Geometry check sheet. Reference: the model listing, model coordinates, mm. Face numbers are marked on the shaded views. A direction names the side the tool comes from. Coordinates: 2 decimals unless noted, no trailing zeros. Loops run counter-clockwise (first coordinate to the right, second up) from the corner with the lowest first, then second, coordinate; pieces in that order, holes last.
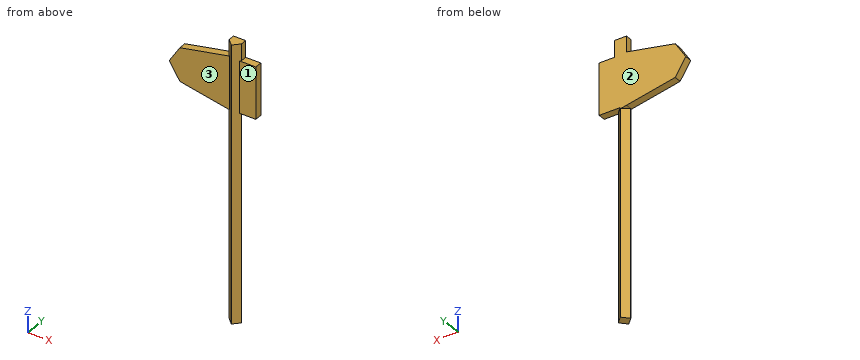
from build123d import *

# Parameters (mm, degrees)
F0_W         = 10.6080286205
F0_H         = 181.0148730874
F1_DEPTH     = 10.52446
F0_W_2       = 13.1920464337
F0_H_2       = 45.1798141003
F2_DEPTH     = 6.38094
F3_T1_DEPTH  = 194.0790226663
F3_T6_DEPTH  = 266.8450713117
F3_T12_DEPTH = 266.8450713117
F3_T18_DEPTH = 266.8450713117
F3_T25_DEPTH = 266.8450713117
F3_T31_DEPTH = 266.8450713117
F3_T37_DEPTH = 266.8450713117
F3_T43_DEPTH = 266.8450713117
F3_T49_DEPTH = 266.8450713117
F3_T56_DEPTH = 266.8450713117
F3_T62_DEPTH = 266.8450713117
F3_T68_DEPTH = 207.1431722451


# Not quite as in the source:
# - a fillet or chamfer that OpenCascade refuses, or shapes differently, is made with other operations: its cross-section is extruded or revolved along the edge and cut away or added


with BuildPart() as f1:
    # F0 (on Front) → F1 (new body)
    with BuildSketch(Plane.XZ):
        with Locations((36.9313266128, -119.8917590082)):
            Rectangle(F0_W, F0_H)
        Polygon((42.2353409231, 15.7954916358), (42.2353409231, 30.3175766021), (31.6273123026, 30.3175766021), (31.6273123026, 16.6022777557), align=None)
        Polygon((42.2353409231, -29.3843224645), (42.2353409231, 15.7954916358), (31.6273123026, 16.6022777557), (31.6273123026, -29.3843224645), align=None)
    extrude(amount=F1_DEPTH)

    # F0 (on Front) → F2 (join)
    with BuildSketch(Plane.XZ):
        Polygon((42.2353409231, 15.7954916358), (42.2353409231, 30.3175766021), (31.6273123026, 30.3175766021), (31.6273123026, 16.6022777557), align=None)
        with Locations((48.8313641399, -6.7944154143)):
            Rectangle(F0_W_2, F0_H_2)
        Polygon((42.2353409231, -29.3843224645), (42.2353409231, 15.7954916358), (31.6273123026, 16.6022777557), (31.6273123026, -29.3843224645), align=None)
        with Locations((36.9313266128, -119.8917590082)):
            Rectangle(F0_W, F0_H)
        Polygon((31.6273123026, -29.3843224645), (31.6273123026, 16.6022777557), (-10.7287643477, 8.1310607493), (-20.0067628175, -6.3910223544), (-10.7287643477, -20.913105458), align=None)
    extrude(amount=F2_DEPTH)

    # F3: chamfer of 5.08 on 4 edges, made by hand

    # F3_s2 → F3_t1 (cut)
    with BuildSketch(Plane.XY.offset(-223.4633451307)):
        Polygon((42.2353409231, -5.08), (37.1553409231, 0), (42.2353409231, 0), align=None)
    extrude(amount=F3_T1_DEPTH, mode=Mode.SUBTRACT)


with BuildPart() as f3_tool4:
    # F3_s5 → F3_t6 (new body)
    with BuildSketch(Plane.XY.offset(-223.4633451307)):
        Polygon((42.2353409231, -5.44446), (37.1553409231, -10.52446), (42.2353409231, -10.52446), align=None)
    extrude(amount=F3_T6_DEPTH)

    split(bisect_by=Plane.XZ.offset(6.38094), keep=Keep.BOTTOM)

    split(bisect_by=Plane.XY.offset(-29.3843224645), keep=Keep.BOTTOM)


with BuildPart() as f1_1:
    add(f1.part)

    # F3_t3: cut F3_tool4
    add(f3_tool4.part, mode=Mode.SUBTRACT)


with BuildPart() as f3_tool10:
    # F3_s11 → F3_t12 (new body)
    with BuildSketch(Plane.XY.offset(-223.4633451307)):
        Polygon((42.2353409231, -5.44446), (37.1553409231, -10.52446), (42.2353409231, -10.52446), align=None)
    extrude(amount=F3_T12_DEPTH)

    split(bisect_by=Plane.XZ.offset(6.38094), keep=Keep.TOP)

    split(bisect_by=Plane.XY.offset(-29.3843224645), keep=Keep.BOTTOM)


with BuildPart() as f1_2:
    add(f1_1.part)

    # F3_t9: cut F3_tool10
    add(f3_tool10.part, mode=Mode.SUBTRACT)


with BuildPart() as f3_tool16:
    # F3_s17 → F3_t18 (new body)
    with BuildSketch(Plane.XY.offset(-223.4633451307)):
        Polygon((42.2353409231, -5.44446), (37.1553409231, -10.52446), (42.2353409231, -10.52446), align=None)
    extrude(amount=F3_T18_DEPTH)

    split(bisect_by=Plane.XY.offset(15.7954916358), keep=Keep.BOTTOM)

    split(bisect_by=Plane.XZ.offset(6.38094), keep=Keep.TOP)

    split(bisect_by=Plane.XY.offset(-29.3843224645), keep=Keep.TOP)


with BuildPart() as f1_3:
    add(f1_2.part)

    # F3_t15: cut F3_tool16
    add(f3_tool16.part, mode=Mode.SUBTRACT)


with BuildPart() as f3_tool23:
    # F3_s24 → F3_t25 (new body)
    with BuildSketch(Plane.XY.offset(-223.4633451307)):
        Polygon((42.2353409231, -5.44446), (37.1553409231, -10.52446), (42.2353409231, -10.52446), align=None)
    extrude(amount=F3_T25_DEPTH)

    split(bisect_by=Plane.XY.offset(15.7954916358), keep=Keep.TOP)

    split(bisect_by=Plane.XZ.offset(6.38094), keep=Keep.BOTTOM)


with BuildPart() as f1_4:
    add(f1_3.part)

    # F3_t22: cut F3_tool23
    add(f3_tool23.part, mode=Mode.SUBTRACT)


with BuildPart() as f3_tool29:
    # F3_s30 → F3_t31 (new body)
    with BuildSketch(Plane.XY.offset(-223.4633451307)):
        Polygon((42.2353409231, -5.44446), (37.1553409231, -10.52446), (42.2353409231, -10.52446), align=None)
    extrude(amount=F3_T31_DEPTH)

    split(bisect_by=Plane.XY.offset(15.7954916358), keep=Keep.TOP)

    split(bisect_by=Plane.XZ.offset(6.38094), keep=Keep.TOP)


with BuildPart() as f1_5:
    add(f1_4.part)

    # F3_t28: cut F3_tool29
    add(f3_tool29.part, mode=Mode.SUBTRACT)


with BuildPart() as f3_tool35:
    # F3_s36 → F3_t37 (new body)
    with BuildSketch(Plane.XY.offset(43.381726181)):
        Polygon((31.6273123026, -5.44446), (36.7073123026, -10.52446), (31.6273123026, -10.52446), align=None)
    extrude(amount=-F3_T37_DEPTH)

    split(bisect_by=Plane.XZ.offset(6.38094), keep=Keep.BOTTOM)

    split(bisect_by=Plane(origin=(-1.976310754, 0, 9.8815518144), x_dir=(0, 1, 0), z_dir=(-0.1961161725, 0, 0.9805806682)), keep=Keep.TOP)


with BuildPart() as f1_6:
    add(f1_5.part)

    # F3_t34: cut F3_tool35
    add(f3_tool35.part, mode=Mode.SUBTRACT)


with BuildPart() as f3_tool41:
    # F3_s42 → F3_t43 (new body)
    with BuildSketch(Plane.XY.offset(43.381726181)):
        Polygon((31.6273123026, -5.44446), (36.7073123026, -10.52446), (31.6273123026, -10.52446), align=None)
    extrude(amount=-F3_T43_DEPTH)

    split(bisect_by=Plane.XZ.offset(6.38094), keep=Keep.TOP)

    split(bisect_by=Plane(origin=(-1.976310754, 0, 9.8815518144), x_dir=(0, 1, 0), z_dir=(-0.1961161725, 0, 0.9805806682)), keep=Keep.TOP)


with BuildPart() as f1_7:
    add(f1_6.part)

    # F3_t40: cut F3_tool41
    add(f3_tool41.part, mode=Mode.SUBTRACT)


with BuildPart() as f3_tool47:
    # F3_s48 → F3_t49 (new body)
    with BuildSketch(Plane.XY.offset(43.381726181)):
        Polygon((31.6273123026, -5.44446), (36.7073123026, -10.52446), (31.6273123026, -10.52446), align=None)
    extrude(amount=-F3_T49_DEPTH)

    split(bisect_by=Plane(origin=(-4.4343967239, 0, -22.1719792319), x_dir=(0, 1, 0), z_dir=(0.1961161725, 0, 0.9805806682)), keep=Keep.TOP)

    split(bisect_by=Plane.XZ.offset(6.38094), keep=Keep.TOP)

    split(bisect_by=Plane(origin=(-1.976310754, 0, 9.8815518144), x_dir=(0, 1, 0), z_dir=(0.1961161725, 0, -0.9805806682)), keep=Keep.TOP)


with BuildPart() as f1_8:
    add(f1_7.part)

    # F3_t46: cut F3_tool47
    add(f3_tool47.part, mode=Mode.SUBTRACT)


with BuildPart() as f3_tool54:
    # F3_s55 → F3_t56 (new body)
    with BuildSketch(Plane.XY.offset(43.381726181)):
        Polygon((31.6273123026, -5.44446), (36.7073123026, -10.52446), (31.6273123026, -10.52446), align=None)
    extrude(amount=-F3_T56_DEPTH)

    split(bisect_by=Plane(origin=(-4.4343967239, 0, -22.1719792319), x_dir=(0, 1, 0), z_dir=(-0.1961161725, 0, -0.9805806682)), keep=Keep.TOP)

    split(bisect_by=Plane.XZ.offset(6.38094), keep=Keep.BOTTOM)


with BuildPart() as f1_9:
    add(f1_8.part)

    # F3_t53: cut F3_tool54
    add(f3_tool54.part, mode=Mode.SUBTRACT)


with BuildPart() as f3_tool60:
    # F3_s61 → F3_t62 (new body)
    with BuildSketch(Plane.XY.offset(43.381726181)):
        Polygon((31.6273123026, -5.44446), (36.7073123026, -10.52446), (31.6273123026, -10.52446), align=None)
    extrude(amount=-F3_T62_DEPTH)

    split(bisect_by=Plane(origin=(-4.4343967239, 0, -22.1719792319), x_dir=(0, 1, 0), z_dir=(-0.1961161725, 0, -0.9805806682)), keep=Keep.TOP)

    split(bisect_by=Plane.XZ.offset(6.38094), keep=Keep.TOP)


with BuildPart() as f1_10:
    add(f1_9.part)

    # F3_t59: cut F3_tool60
    add(f3_tool60.part, mode=Mode.SUBTRACT)


with BuildPart() as f3_tool66:
    # F3_s67 → F3_t68 (new body)
    with BuildSketch(Plane.XY.offset(-16.3201728856)):
        Polygon((31.6273123026, -5.08), (36.7073123026, 0), (31.6273123026, 0), align=None)
    extrude(amount=-F3_T68_DEPTH)

    split(bisect_by=Plane(origin=(-4.4343967239, 0, -22.1719792319), x_dir=(0, 1, 0), z_dir=(-0.1961161725, 0, -0.9805806682)), keep=Keep.TOP)


with BuildPart() as f1_11:
    add(f1_10.part)

    # F3_t65: cut F3_tool66
    add(f3_tool66.part, mode=Mode.SUBTRACT)


solid = f1_11.part
(1) Gauge pin test, flat ends, axial feed: pin 1 Ø6 at (y, z) = (-3.5, -118.5) entering from +X; pin 2 Ø1.5 at (x, y) = (29.5, -6) entering from +Z; pin 3 Ø4 at (y, z) = (-2.5, -76.5) entering from +X. Record the tip position at first contact, or that the pin passes through.
Findings:
pin 1: stops at x = 42.24
pin 2: stops at z = 16.33
pin 3: stops at x = 41.66
(2) Sectioned sample at A-A on z = -51.5. Record the cut outline in (x, y).
Findings:
outline: (31.63, -5.44) - (36.71, -10.52) - (37.16, -10.52) - (42.24, -5.44) - (42.24, -5.08) - (37.16, 0) - (36.71, 0) - (31.63, -5.08) - close
(3) Sectioned sample at D-D on z = -17. Record the cut outline in (x, y).
Findings:
outline: (-13.23, -6.38) - (32.56, -6.38) - (36.71, -10.52) - (37.16, -10.52) - (41.3, -6.38) - (55.43, -6.38) - (55.43, 0) - (-13.23, 0) - close
(4) Scan lines: L1, parallel to Z at x = 50.5, y = -0.25; L2, parallel to X at y = -8, z = -122; L3, parallel to Z at x = 3, y = -5.75. Record each from-to range of solid material in increasing order.
Findings:
L1: z = -29.38 to 15.8
L2: x = 34.18 to 39.68
L3: z = -23.66 to 10.88
(5) Access from +Z, -Z, +X, -X, +Y, -Y to the whole of each face (thin tool, end or side, straight path). Record for the marked faces 1, 2 and 3.
Findings:
face 1: +Z, -Z, +X, -Y
face 2: +Z, -Z, +X, -X, +Y
face 3: +Z, -Z, -X, -Y
(6) Sectioned sample at B-B on x = 50. Record the cut outline in (y, z).
Findings:
outline: (-6.38, -29.38) - (0, -29.38) - (0, 15.8) - (-6.38, 15.8) - close
(7) Sectioned sample at C-C on y = -2. Record the cut outline in (x, z).
Findings:
outline: (-20.01, -6.39) - (-10.73, -20.91) - (34.71, -30) - (34.71, -210.4) - (39.16, -210.4) - (39.16, -29.38) - (55.43, -29.38) - (55.43, 15.8) - (42.24, 15.8) - (42.24, 30.32) - (31.63, 30.32) - (31.63, 16.6) - (-10.73, 8.13) - close
